Geometry check sheet. Reference: drawing and pictorial views, mm from the part's lowest x, y, z. A direction names the side the tool comes from. Coordinates: 2 decimals unless noted, no trailing zeros. Write each loop counter-clockwise with the first axis right and the second up, starting at its lowest first coordinate (ties: lowest second). Pieces come first, ordered by that corner, then holes. Notation, with made-up numbers: (78, -23) -> (123, -23) arc R11 cw to (123, -19) -> close; hole circle Ø1 at (65.25, -6). An arc over 180 degrees is marked (long way). Put each result on its own line as item: value.
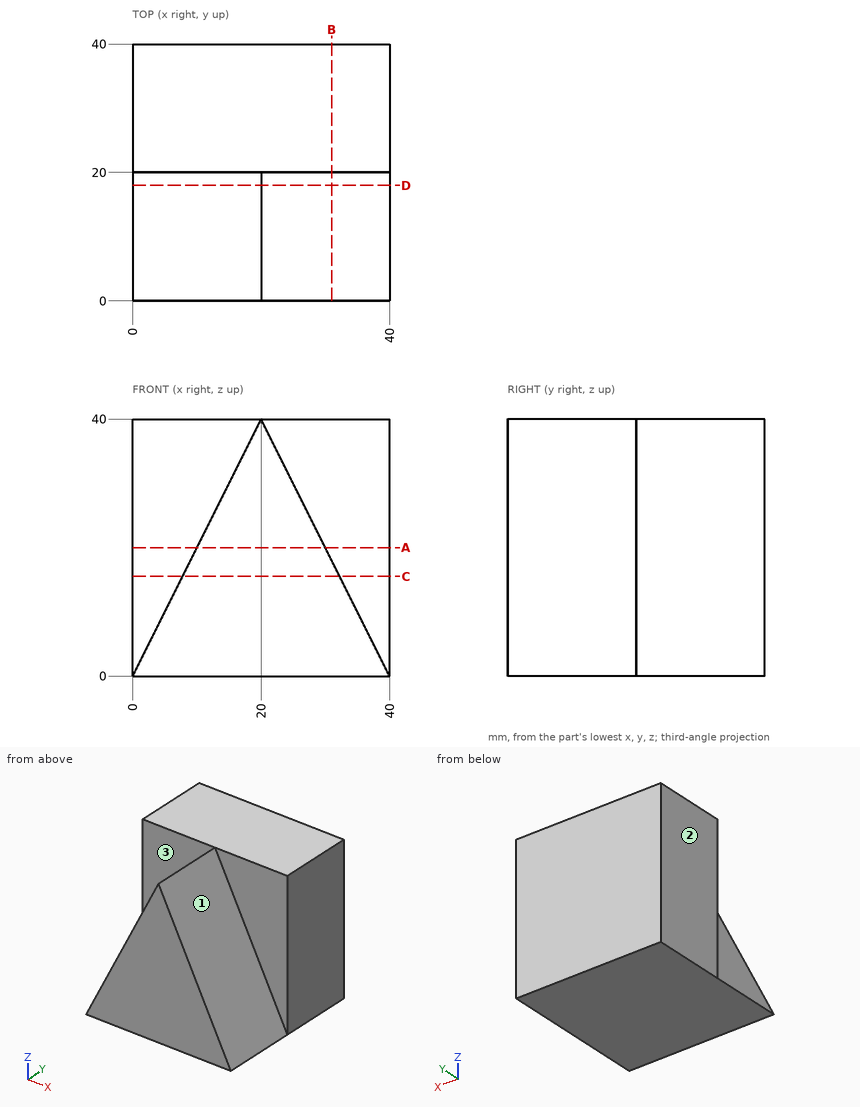
Q1. Cross-section at B-B (x = 31). Record the cut outline in (y, z).
Recorded:
outline: (0, 0) -> (40, 0) -> (40, 40) -> (20, 40) -> (20, 18) -> (0, 18) -> close
Q2. Cross-section at D-D (y = 18). Record the cut outline in (x, z).
Recorded:
outline: (0, 0) -> (40, 0) -> (20, 40) -> close
Q3. Tool access check on the marked faces 1, 2 and 3. Record the directions out of +Z, -Z, +X, -X, +Y, -Y that give a thin tool (end or side, any length) a straight path to the whole face; none if there is none.
Recorded:
face 1: +Z, +X, -Y
face 2: +Z, -Z, -X, +Y, -Y
face 3: +Z, -X, -Y
Q4. Cross-section at A-A (z = 20). Record the cut outline in (x, y).
Recorded:
outline: (0, 20) -> (10, 20) -> (10, 0) -> (30, 0) -> (30, 20) -> (40, 20) -> (40, 40) -> (0, 40) -> close
Q5. Cross-section at C-C (z = 15.5). Record the cut outline in (x, y).
Recorded:
outline: (0, 20) -> (7.75, 20) -> (7.75, 0) -> (32.25, 0) -> (32.25, 20) -> (40, 20) -> (40, 40) -> (0, 40) -> close
Q6. Depth check by flat-ended pin: P1, Ø4, axis at x = 6, y = 9.5, coming from the +Z side; P2, Ø4, axis at y = 17, z = 16, coming from the +X side; P3, Ø3, axis at y = 11, z = 13.5, coming from the -X side. Enter the tip coordinate at first touch or a pass-through.
Recorded:
P1: stops at z = 16
P2: stops at x = 33
P3: stops at x = 6
Q7. Material ranges on line 1 along Y through (x, z) = (38, 32); line 2 along X through (y, z) = (12, 13); line 3 along X through (y, z) = (10, 22), recorded low to high.
Recorded:
line 1: y = 20 to 40
line 2: x = 6.5 to 33.5
line 3: x = 11 to 29
